Design review of the part shown in the three views and the two pictorial views. Dimensions are in mm from the part's minimum x, y and z. A direction names the side the tool comes from. Coordinates: 2 decimals unless noted, no trailing zeros. Order: outer loops, then holes, each group sorted by start corner. A loop starts at its lowest first (then second) coordinate and runs counter-clockwise, first axis right, second up. Notation, with made-up numbers: (44.5, 73.25) -> (76.5, 73.25) arc R20 cw to (76.5, 111.25) -> close; hole circle Ø7 at (-30, 78.25). An arc over 180 degrees is marked (long way). Write item = value, one per line. Start each with the question number.
1) Machinability: for the marked faces 1 and 2, which of the approach directions +Z, -Z, +X, -X, +Y, -Y give a long, thin tool a straight path to every point of the face, cutting with its end or side? Answer none if there is none.
2) Consider section A-A on x = 5. Give the boundary of the cut face in (y, z).
3) Consider section B-B on z = 5. Give the boundary of the cut face in (x, y), and give its area (3 significant figures).
4) Wall thickness on probe 1 along X at (y, z) = (19, 6.25); probe 2 along Z at (x, y) = (2.75, 13.5): over which ranges is each line inside the solid? List them lowest first. Write a range as [from, to].
5) Consider section C-C on y = 12. Give the boundary of the cut face in (x, z).
6) Draft analysis for pull direction Z (two halves, no side actions). For the marked faces 3, 4, 5 and 6, state which applies: +Z half, -Z half, draft (parallel to the pull), parting line (faces both ways), or undercut.
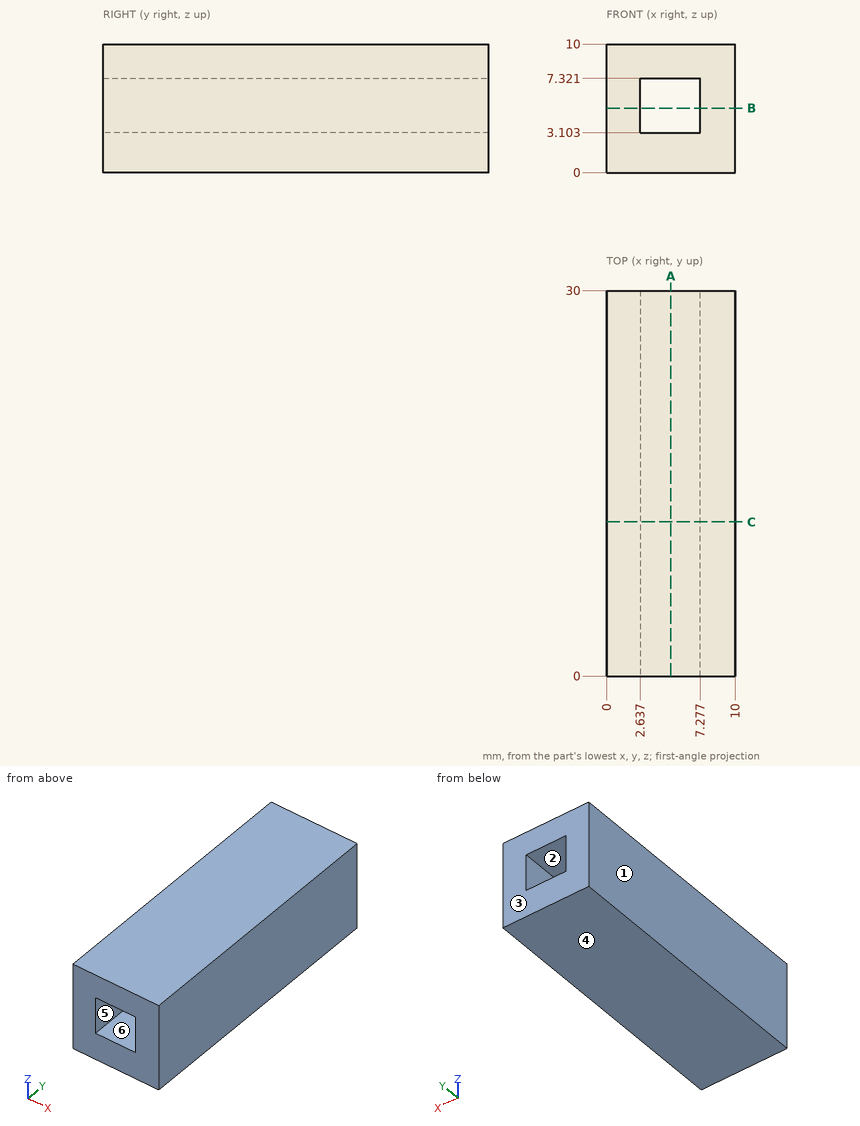
Answer sheet:
q1.face_1 = +Z, -Z, -X, +Y, -Y
q1.face_2 = +Y, -Y
q2.outline = (0, 0) -> (30, 0) -> (30, 3.1) -> (0, 3.1) -> close; (0, 7.32) -> (30, 7.32) -> (30, 10) -> (0, 10) -> close
q3.outline = (0, 0) -> (2.64, 0) -> (2.64, 30) -> (0, 30) -> close; (7.28, 0) -> (10, 0) -> (10, 30) -> (7.28, 30) -> close
q3.area = 161 mm2
q4.probe_1 = [0, 2.64], [7.28, 10]
q4.probe_2 = [0, 3.1], [7.32, 10]
q5.outline = (0, 0) -> (10, 0) -> (10, 10) -> (0, 10) -> close; hole (2.64, 3.1) -> (7.28, 3.1) -> (7.28, 7.32) -> (2.64, 7.32) -> close
q6.face_3 = draft
q6.face_4 = -Z half
q6.face_5 = undercut
q6.face_6 = undercut
